Read the model definition and answer for the solid it produces. Units are mm, in the model's axes. Face numbers are marked on the shaded views. A direction names the side the tool comes from. Coordinates: 2 decimals unless noted, no trailing zeros. Order: outer loops, then holes, each group sorted by start corner. A loop starts at its lowest first (then second) coordinate and runs counter-clockwise, first axis right, second up. Notation, with made-up numbers: M 51,-9 L 106,-9 A18 ccw 106,-3 Z; hole C 24.5,-32.75 d9. An arc over 180 degrees is marked long. Use a Markdown table: item, result. Add a question column.
1) Find the intervals of material crossed by probe 1 along X at (y, z) = (1, -3); probe 2 along X at (y, z) = (-1.5, -13.5); probe 3 along Z at (x, y) = (9.75, 1), in increasing order. Write a range as [from, to].
2) The mould has two halves that part along X. Classify the marked faces 4, 5, 6 and 7: released by +X, released by -X, zero draft, split by the parting line, or undercut.
3) Find section D-D on x = 7.75. Write down the section's boundary in (y, z).
4) Find section A-A on z = -3. Write down the section's boundary in (x, y), plus the area to 3 significant figures.
5) Find section B-B on z = -13. Write down the section's boundary in (x, y), plus the area to 4 significant figures.
6) Find section C-C on y = 2. Count the separate pieces of the cut face and the enclosed holes in it, plus the area to 3 significant figures.
7) Each of these flat-tipped pins is pushed along its axis until it touches: pin 1 Ø3 at (y, z) = (3.5, -13) entering from -X; pin 2 Ø4 at (x, z) = (9, -5.5) entering from +Y; pin 3 Ø2.5 at (x, z) = (14.5, -3) entering from -Y; pin 4 Ø0.9 at (x, y) = (7, 4) entering from +Z. Where does it stop, or does it pass through?
8) For the marked faces 1, 2 and 3, determine the directions among +Z, -Z, +X, -X, +Y, -Y from which every point of the face is accessible in a straight line to the end or side of a thin tool.
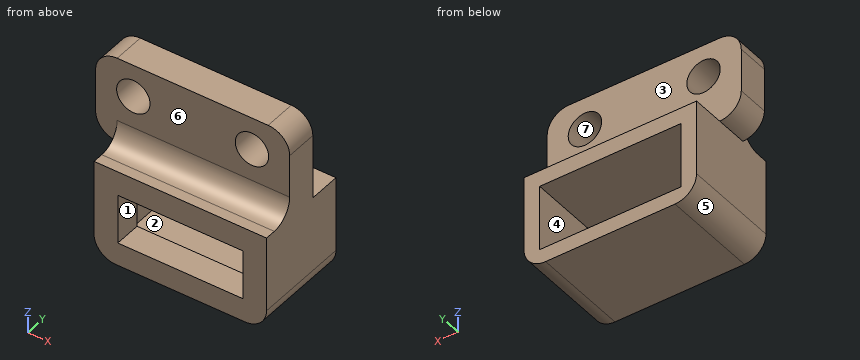
from build123d import *

# Parameters (mm, degrees)
CROQUIS1_W              = 18
CROQUIS1_H              = 18
CROQUIS1_R              = 1.55
SALIENTE_EXTRUIR1_DEPTH = 3
CROQUIS3_W              = 18
CROQUIS3_H              = 10
SALIENTE_EXTRUIR3_DEPTH = 3
CORTAR_EXTRUIR1_REACH   = 28.153
CROQUIS4_W              = 2
CROQUIS4_H              = 10
CROQUIS7_W              = 13.1
CROQUIS7_H              = 6.1
CORTAR_EXTRUIR2_DEPTH   = 6
CROQUIS9_W              = 16
CROQUIS9_H              = 10
CROQUIS9_W_2            = 13.1
CROQUIS9_H_2            = 6.1
SALIENTE_EXTRUIR4_DEPTH = 3
CROQUIS10_W             = 13.1
CROQUIS10_H             = 6.1
CROQUIS10_W_2           = 11.6
CROQUIS10_H_2           = 4.6
SALIENTE_EXTRUIR6_DEPTH = 2.5
CROQUIS11_W             = 16
CROQUIS11_H             = 1
CORTAR_EXTRUIR4_DEPTH   = 9
REDONDEO1_R             = 2


with BuildPart() as part:
    # Croquis1 → Saliente-Extruir1 (new body)
    with BuildSketch(Plane(origin=(0, 0, 0), x_dir=(1, 0, 0), z_dir=(0, 1, 0))):
        with Locations((9, 9)):
            Rectangle(CROQUIS1_W, CROQUIS1_H)
        with Locations(Location((3.5, 3, 0), (0, 0, 270))):
            Circle(CROQUIS1_R, mode=Mode.SUBTRACT)
        with Locations(Location((14.5, 3, 0), (0, 0, 270))):
            Circle(CROQUIS1_R, mode=Mode.SUBTRACT)
    extrude(amount=SALIENTE_EXTRUIR1_DEPTH)

    # Croquis3 → Saliente-Extruir3 (add)
    with BuildSketch(Plane(origin=(0, 3, 0), x_dir=(1, 0, 0), z_dir=(0, 1, 0))):
        with Locations((9, 13)):
            Rectangle(CROQUIS3_W, CROQUIS3_H)
    extrude(amount=SALIENTE_EXTRUIR3_DEPTH)

    # Cortar-Extruir1: up to this face of the body (flat: up to its plane)
    cortar_extruir1_end = Plane(part.part.faces().sort_by_distance((9, 6, -13))[0])
    # Croquis4 → Cortar-Extruir1 (cut, up to the picked face)
    with BuildSketch(Plane.XZ, mode=Mode.PRIVATE) as cortar_extruir1_sk1:
        with Locations((1, -13)):
            Rectangle(CROQUIS4_W, CROQUIS4_H)
    cortar_extruir1_tool1 = split(extrude(cortar_extruir1_sk1.sketch, amount=-CORTAR_EXTRUIR1_REACH, mode=Mode.PRIVATE), bisect_by=cortar_extruir1_end, keep=Keep.BOTH, mode=Mode.PRIVATE)
    add(cortar_extruir1_tool1.solids().sort_by(Axis((1, 0, -13), (0, 1, 0)))[0], mode=Mode.SUBTRACT)

    # Croquis7 → Cortar-Extruir2 (cut)
    with BuildSketch(Plane(origin=(0, 6, 0), x_dir=(1, 0, 0), z_dir=(0, 1, 0))):
        with Locations((10, 12.55)):
            Rectangle(CROQUIS7_W, CROQUIS7_H)
    extrude(amount=-CORTAR_EXTRUIR2_DEPTH, mode=Mode.SUBTRACT)

    # Croquis9 → Saliente-Extruir4 (add)
    with BuildSketch(Plane.XZ):
        with Locations((10, -13)):
            Rectangle(CROQUIS9_W, CROQUIS9_H)
        with Locations((10, -12.55)):
            Rectangle(CROQUIS9_W_2, CROQUIS9_H_2, mode=Mode.SUBTRACT)
    extrude(amount=SALIENTE_EXTRUIR4_DEPTH)

    # Croquis10 → Saliente-Extruir6 (add)
    with BuildSketch(Plane.XZ.offset(3)):
        with Locations((10, -12.55)):
            Rectangle(CROQUIS10_W, CROQUIS10_H)
        with Locations((10, -12.55)):
            Rectangle(CROQUIS10_W_2, CROQUIS10_H_2, mode=Mode.SUBTRACT)
    extrude(amount=-SALIENTE_EXTRUIR6_DEPTH)

    # Croquis11 → Cortar-Extruir4 (cut)
    with BuildSketch(Plane(origin=(0, 6, 0), x_dir=(1, 0, 0), z_dir=(0, 1, 0))):
        with Locations((10, 17.5)):
            Rectangle(CROQUIS11_W, CROQUIS11_H)
    extrude(amount=-CORTAR_EXTRUIR4_DEPTH, mode=Mode.SUBTRACT)

    # Redondeo1
    redondeo1_edges = [part.edges().sort_by_distance(p)[0] for p in [
        (10, 0, -8),
    ]]
    fillet(redondeo1_edges, radius=REDONDEO1_R)
    redondeo1_2_edges = [part.edges().sort_by_distance(p)[0] for p in [
        (18, 1.5, -17),
        (2, 1.5, -17),
        (0, 1.5, -8),
        (18, 1.5, 0),
        (0, 1.5, 0),
    ]]
    fillet(redondeo1_2_edges, radius=REDONDEO1_R - 0.0001)  # a hair under: the kernel refuses the full size


solid = part.part
Check result:
| question | item | result |
|---|---|---|
| 1 | probe 1 | x = [0, 1.95], [5.05, 12.95], [16.05, 18] |
| 1 | probe 2 | x = [2, 4.2], [15.8, 18] |
| 1 | probe 3 | z = [-17, -15.6], [-9.5, 0] |
| 2 | face 4 | undercut |
| 2 | face 5 | released by -X |
| 2 | face 6 | zero draft |
| 2 | face 7 | undercut |
| 3 | outline | M -3,-17 L 6,-17 L 6,-15.6 L -0.5,-15.6 L -0.5,-14.85 L -3,-14.85 Z; M -3,-10.25 L -0.5,-10.25 L -0.5,-9.5 L 6,-9.5 L 6,-8 L 3,-8 L 3,0 L 0,0 L 0,-6 A2 cw -2,-8 L -3,-8 Z |
| 4 | outline | M 0,0 L 1.95,0 L 1.95,3 L 0,3 Z; M 5.05,0 L 12.95,0 L 12.95,3 L 5.05,3 Z; M 16.05,0 L 18,0 L 18,3 L 16.05,3 Z |
| 4 | area | 35.4 mm2 |
| 5 | outline | M 2,-3 L 4.2,-3 L 4.2,-0.5 L 3.45,-0.5 L 3.45,6 L 2,6 Z; M 15.8,-3 L 18,-3 L 18,6 L 16.55,6 L 16.55,-0.5 L 15.8,-0.5 Z |
| 5 | area | 29.85 mm2 |
| 6 | separate pieces | 1 |
| 6 | enclosed holes | 3 |
| 6 | area | 189 mm2 |
| 7 | pin 1 | stops at x = 2 |
| 7 | pin 2 | stops at y = 3 |
| 7 | pin 3 | passes through |
| 7 | pin 4 | stops at z = -8 |
| 8 | face 1 | +Y, -Y |
| 8 | face 2 | +Y |
| 8 | face 3 | +Z, +X, -X, +Y |
